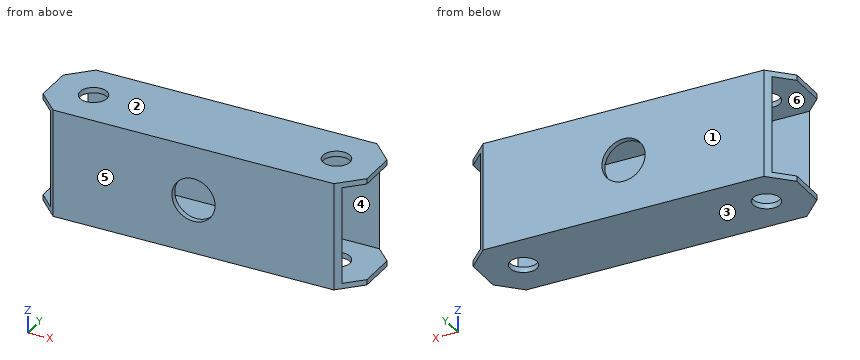
from build123d import *

# Parameters (mm, degrees)
SKETCH1_W           = 120
SKETCH1_H           = 40
BOSS_EXTRUDE3_DEPTH = 30
SKETCH3_R           = 5
CUT_EXTRUDE2_DEPTH  = 131
CUT_EXTRUDE3_DEPTH  = 120
SKETCH6_R           = 8
CUT_EXTRUDE4_DEPTH  = 120
CHAMFER2_SIZE       = 8


with BuildPart() as part:
    # Sketch1 → Boss-Extrude3 (new body)
    with BuildSketch(Plane(origin=(0, 0, 0), x_dir=(1, 0, 0), z_dir=(0, 1, 0))):
        with Locations((60, 20)):
            Rectangle(SKETCH1_W, SKETCH1_H)
    extrude(amount=BOSS_EXTRUDE3_DEPTH)

    # Sketch3 → Cut-Extrude2 (cut, through all)
    with BuildSketch(Plane(origin=(0, 0, -40), x_dir=(-1, 0, 0), z_dir=(0, 0, -1))):
        with Locations((-105, 15)):
            Circle(SKETCH3_R)
        with Locations(Location((-15, 15, 0), (0, 0, 180))):
            Circle(SKETCH3_R)
    extrude(amount=-CUT_EXTRUDE2_DEPTH, mode=Mode.SUBTRACT)

    # 3DSketch1 → Cut-Extrude3 (cut)
    with BuildSketch(Plane(origin=(0, 28, -2), x_dir=(0, -0.5854905538443583, -0.8106792283998812), z_dir=(-1, 0, 0))):
        Polygon((0, 0), (29.184452222, -21.077659938), (44.407206622, 0), (15.2227544, 21.077659938), align=None)
    extrude(amount=-CUT_EXTRUDE3_DEPTH, mode=Mode.SUBTRACT)

    # Sketch6 → Cut-Extrude4 (cut)
    with BuildSketch(Plane(origin=(0, 30, 0), x_dir=(1, 0, 0), z_dir=(0, 1, 0))):
        with Locations(Location((60, 20, 0), (0, 0, 270))):
            Circle(SKETCH6_R)
    extrude(amount=-CUT_EXTRUDE4_DEPTH, mode=Mode.SUBTRACT)

    # Chamfer2
    # the kernel refuses this chamfer: 8 mm, written as the material it takes off along each edge
    with BuildSketch(Plane(origin=(0, 0, -60.573463904), x_dir=(-0.027495876610586372, 0.9996219169112968, 0), z_dir=(0, 0, 1)), Plane(origin=(120, 30, 20.573463904), x_dir=(-0.9996219169112968, 0.02749587661058651, 0), z_dir=(0, 0, -1))) as chamfer2_piece_1:
        Polygon((CHAMFER2_SIZE * 0.999621916911, -CHAMFER2_SIZE * 0.0274958766106), (-CHAMFER2_SIZE * 0.0274958766106, -CHAMFER2_SIZE * 0.999621916911), (0, 0), align=None)
    extrude(amount=81.146927807, mode=Mode.SUBTRACT)
    with BuildSketch(Plane(origin=(0, 30, -60.573463904), x_dir=(-0.027495876610586365, -0.9996219169112968, 0), z_dir=(0, 0, 1)), Plane(origin=(120, 0, 20.573463904), x_dir=(-0.9996219169112968, -0.02749587661058639, 0), z_dir=(0, 0, -1))) as chamfer2_piece_2:
        Polygon((CHAMFER2_SIZE * 0.999621916911, CHAMFER2_SIZE * 0.0274958766106), (-CHAMFER2_SIZE * 0.0274958766106, CHAMFER2_SIZE * 0.999621916911), (0, 0), align=None)
    extrude(amount=81.146927807, mode=Mode.SUBTRACT)


solid = part.part
Check sheet for the modelled part. Datum: model origin and axes. Units: mm. Face numbers are marked on the shaded views. A direction names the side the tool comes from. Round coordinates to 2 decimals unless told otherwise and drop trailing zeros. Order: outer loops, then holes, each group sorted by start corner. A loop starts at its lowest first (then second) coordinate and runs counter-clockwise, first axis right, second up. Notation, with made-up numbers: M 85.5,11 L 112.5,11 A31 ccw 112.5,39 Z; hole C 27,20 d3. An arc over 180 degrees is marked long. One line per item, written item: value. Start each with the question number.
1. Section check D-D on z = -20. Enter the section's corners in (x, y), and give its area (3 significant figures).
2. Release check for a two-part mould opening along Z. For the marked faces 1, 2, 3 and 4 record: released by +Z, released by -Z, zero draft, split by the parting line, or undercut.
3. Access from +Z, -Z, +X, -X, +Y, -Y to the whole of each face (thin tool, end or side, straight path). Record for the marked faces 5 and 6.
4. Section check B-B on z = -32. Enter the section's corners in (x, y), and give its area (3 significant figures).
5. Section check C-C on x = 60. Enter the section's corners in (y, z).
6. Section check A-A on y = 15. Enter the section's corners in (x, z), and give its area (3 significant figures).
7. Gauge pin test, flat ends, axial feed: P1, Ø13, axis at x = 60, z = -20, coming from the +Y side; P2, Ø4, axis at y = 3.5, z = -24.5, coming from the +X side. Record the tip position at first contact, or that the pin passes through.
8. Scan lines: line 1 along Z through (x, y) = (48.5, 18.5); line 2 along Y through (x, z) = (40, -20); line 3 along Y through (x, z) = (105, -39). Record each from-to range of solid material in increasing order.
Results found:
1. outline: M 6,2 L 8,0 L 52,0 L 52,2 Z; M 6,28 L 52,28 L 52,30 L 8,30 Z; M 68,0 L 112,0 L 114,2 L 68,2 Z; M 68,28 L 114,28 L 112,30 L 68,30 Z
1. area: 360 mm^2
2. face 1: zero draft
2. face 2: released by +Z
2. face 3: released by -Z
2. face 4: undercut
3. face 5: +Z, -Z, +X, -X, -Y
3. face 6: +X, -X
4. outline: M 6,2 L 8,0 L 112,0 L 114,2 Z; M 6,28 L 114,28 L 112,30 L 8,30 Z
4. area: 424 mm^2
5. outline: M 0,-40 L 30,-40 L 30,-28 L 28,-28 L 28,-38 L 2,-38 L 2,-28 L 0,-28 Z; M 0,-12 L 2,-12 L 2,-2 L 28,-2 L 28,-12 L 30,-12 L 30,0 L 0,0 Z
6. outline: M 0,-40 L 10,-40 L 10,-38 L 0,-38 Z; M 0,-2 L 10,-2 L 10,0 L 0,0 Z; M 20,-40 L 100,-40 L 100,-38 L 20,-38 Z; M 20,-2 L 100,-2 L 100,0 L 20,0 Z; M 110,-40 L 120,-40 L 120,-38 L 110,-38 Z; M 110,-2 L 120,-2 L 120,0 L 110,0 Z
6. area: 400 mm^2
7. P1: through
7. P2: x = 114
8. line 1: -40 to -38, -2 to 0
8. line 2: 0 to 2, 28 to 30
8. line 3: 0 to 10, 20 to 30
